For this review, take the finished solid that the model builds, in its own axes (mm). Round coordinates to 2 decimals unless told otherwise and drop trailing zeros. Order: outer loops, then holes, each group sorted by start corner. A loop starts at its lowest first (then second) coordinate and runs counter-clockwise, first axis right, second up. Notation, with made-up numbers: (-19, 47) - (35, 47) arc R28 ccw to (35, 73) - close; hole circle Ø6 at (36.25, 74). An arc over 180 degrees is marked (long way). One line per question, with ' | ' between items.
```python
from build123d import *

# Parameters (mm, degrees)
BOSS_EXTRUDE1_DEPTH = 40
FILLET1_R           = 0.5


with BuildPart() as part:
    # Sketch1 → Boss-Extrude1 (new body)
    with BuildSketch(Plane(origin=(0, 0, 0), x_dir=(-1, 0, 0), z_dir=(0, 1, 0))):
        Polygon((-0.376890979, 0.083720177), (8.363244284, -26.866668495), (-29.537452899, -27.083722916), (-38.277588162, -0.133334243), align=None)
    extrude(amount=BOSS_EXTRUDE1_DEPTH)

    # Fillet1
    fillet1_edges = [part.edges().sort_by_distance(p)[0] for p in [
        (10.587104308, 40, -26.975195705),
        (-3.993176653, 40, -13.391474159),
        (19.32723957, 40, -0.024807033),
        (-3.993176653, 0, -13.391474159),
        (10.587104308, 0, -26.975195705),
        (33.907520531, 0, -13.608528579),
        (19.32723957, 0, -0.024807033),
        (33.907520531, 40, -13.608528579),
    ]]
    fillet(fillet1_edges, radius=FILLET1_R)


solid = part.part
```
(1) For probe 1 along Y at (x, z) = (-2.5, -10.25); probe 2 along Z at (x, y) = (12, 15.5); probe 3 along X at (y, z) = (28.5, -4.75), list the stretches that pass through material, from the lowest coordinate up. Write a range as [from, to].
Output values:
probe 1: [0, 40] | probe 2: [-26.98, 0.02] | probe 3: [-1.19, 36.78]
(2) Insertion check: pin 1 (2 mm diameter, centred on y = 22.5, z = -22, fed in from +X); pin 2 (2 mm diameter, centred on x = 11.5, y = 7.5, fed in from -Z); pin 3 (6 mm diameter, centred on y = 10, z = -17, fed in from -X). Each pin has a flat end and moves straight along its axis. Give the tip position at first contact, or say it passes through.
Output values:
pin 1: x = 31.51 | pin 2: z = -26.99 | pin 3: x = -6.14
(3) We need section A-A on y = 13. State the section outline as (x, z) points, plus the area to 3 significant figures.
Output values:
outline: (-8.36, -26.87) - (29.54, -27.08) - (38.28, -0.13) - (0.38, 0.08) - close | area: 1,020 mm^2
